Part model, mm, in its own coordinate system. Face numbers are marked on the shaded views. A direction names the side the tool comes from. Round coordinates to 2 decimals unless told otherwise and drop trailing zeros. Loops run counter-clockwise (first coordinate to the right, second up) from the corner with the lowest first, then second, coordinate; pieces in that order, holes last. Notation, with made-up numbers: (25.25, 84.25) -> (55.25, 84.25) arc R32 cw to (55.25, 110.25) -> close; hole circle Ø1 at (29, 74). An arc over 180 degrees is marked (long way). Use a Markdown table: item, result. Add a question column.
Item 1: Flat gauge pins, fed straight in: pin 1 (10 mm diameter, centred on x = 12, y = 16.5, fed in from -Z); pin 2 (1 mm diameter, centred on x = 0, z = 4.5, fed in from -Y). Where does each tip first touch, or does it go through?
Item 2: Cut at B-B, the plane z = 2.25. List the corners of the cut face in (x, y).
Item 3: Cut at D-D, the plane z = 8.5. List the corners of the cut face in (x, y).
Item 4: Two-plate mould, pull along X, no slides. Class the marked faces 1, 2 and 3: pulls with the +X half, pulls with the -X half, needs draft (parallel to the pull), parting line crosses it, or undercut.
Item 5: Which spindle directions (+Z, -Z, +X, -X, +Y, -Y) get a long thin tool onto all of the face, cutting with end or side? Do the marked faces 4, 5 and 6. Say none if no direction does.
Item 6: Probe line 1 (Y direction, x = 18.5, z = 6); line 2 (Y direction, x = 21, z = 2.75). List the from-to ranges inside material, lowest first. Write a range as [from, to].
Item 7: Cut at A-A, the plane y = -6.5. List the corners of the cut face in (x, z).
```python
from build123d import *

# Parameters (mm, degrees)
F0_W     = 63.5
F0_H     = 63.5
F0_W_2   = 38.1
F0_H_2   = 38.1
F1_DEPTH = 12.7
F2_SIZE  = 5.08
F3_SIZE  = 5.08


with BuildPart() as f1:
    # F0 (on Top) → F1 (new body)
    with BuildSketch(Plane.XY):
        Rectangle(F0_W, F0_H)
        Rectangle(F0_W_2, F0_H_2, mode=Mode.SUBTRACT)
    extrude(amount=F1_DEPTH)

    # F2
    f2_edges = [f1.edges().sort_by_distance(p)[0] for p in [
        (19.05, 0, 0),
        (0, 19.05, 0),
        (-19.05, 0, 0),
        (0, -19.05, 0),
    ]]
    chamfer(f2_edges, length=F2_SIZE)

    # F3
    f3_edges = [f1.edges().sort_by_distance(p)[0] for p in [
        (0, 31.75, 0),
        (-31.75, 0, 0),
        (0, -31.75, 0),
        (31.75, 0, 0),
    ]]
    chamfer(f3_edges, length=F3_SIZE)


solid = f1.part
```
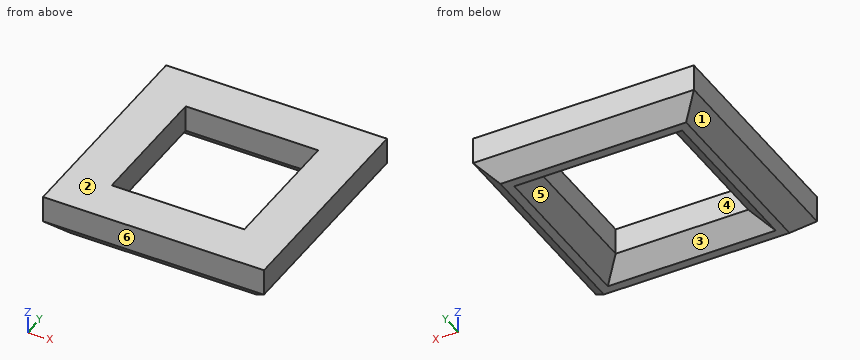
A:
| question | item | result |
|---|---|---|
| 1 | pin 1 | stops at z = 2.63 |
| 1 | pin 2 | stops at y = -31.67 |
| 2 | outline | (-28.92, -28.92) -> (28.92, -28.92) -> (28.92, 28.92) -> (-28.92, 28.92) -> close; hole (-21.88, -21.88) -> (21.88, -21.88) -> (21.88, 21.88) -> (-21.88, 21.88) -> close |
| 3 | outline | (-31.75, -31.75) -> (31.75, -31.75) -> (31.75, 31.75) -> (-31.75, 31.75) -> close; hole (-19.05, -19.05) -> (19.05, -19.05) -> (19.05, 19.05) -> (-19.05, 19.05) -> close |
| 4 | face 1 | pulls with the -X half |
| 4 | face 2 | needs draft |
| 4 | face 3 | undercut |
| 5 | face 4 | +Z, -Z |
| 5 | face 5 | -Z |
| 5 | face 6 | +Z, -Z, +X, -X, -Y |
| 6 | line 1 | y = [-31.75, -19.05], [19.05, 31.75] |
| 6 | line 2 | y = [-29.42, -21.38], [21.38, 29.42] |
| 7 | outline | (-31.75, 5.08) -> (-26.67, 0) -> (-24.13, 0) -> (-19.05, 5.08) -> (-19.05, 12.7) -> (-31.75, 12.7) -> close; (19.05, 5.08) -> (24.13, 0) -> (26.67, 0) -> (31.75, 5.08) -> (31.75, 12.7) -> (19.05, 12.7) -> close |
